Geometry: final body of the model. Coordinates: model frame, mm. Give positions to 0.01 mm unless a question says otherwise; leave off trailing zeros. Write each loop counter-clockwise with the first axis right and the second up, starting at its lowest first coordinate (ties: lowest second). Pieces come first, ordered by that corner, then holes. Notation, with made-up numbers: (48, 20) -> (98, 20) arc R24 cw to (98, 32) -> close; hole circle Ø4 at (-6.75, 88.5). An arc over 180 degrees is marked (long way). Answer as a JSON object with one key per item and string values.
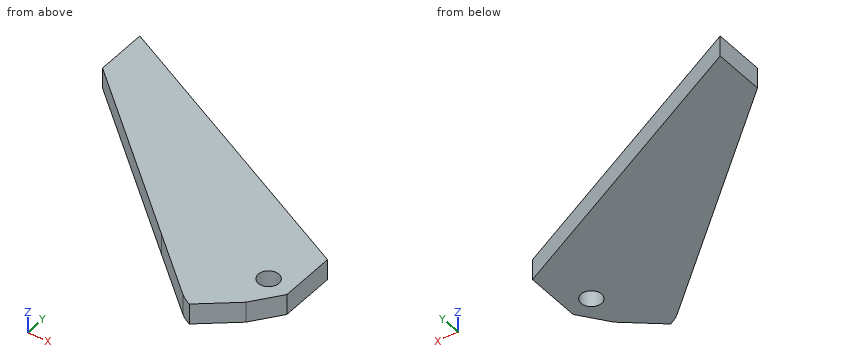
from build123d import *

# Parameters (mm, degrees)
SKETCH1_R           = 1.5
BOSS_EXTRUDE1_DEPTH = 3
CUT_EXTRUDE1_DEPTH  = 3


with BuildPart() as part:
    # Sketch1 → Boss-Extrude1 (new body)
    with BuildSketch(Plane.XY):
        with BuildLine():
            Line((2, 15), (2, 4.201633911))
            ThreePointArc((2, 4.201633911), (-1.543579693, -1.272486957), (-7.988666425, -0.280613309))
            Line((-7.988666425, -0.280613309), (-16.754941475, 7.52032788))
            Line((-16.754941475, 7.52032788), (-40.754941475, 28.877470737))
            Line((-40.754941475, 28.877470737), (-40.754941475, 36.377470737))
            Line((-40.754941475, 36.377470737), (2, 15))
        make_face()
        with Locations((-1.5, 8)):
            Circle(SKETCH1_R, mode=Mode.SUBTRACT)
    extrude(amount=BOSS_EXTRUDE1_DEPTH)

    # Sketch2 → Cut-Extrude1 (cut)
    with BuildSketch(Plane.XY.offset(3)):
        Polygon((-1.061667456, 2.832415464), (-6.529971665, -1.578677992), (-7.079129118, -3.627506614), (6.602158547, -3.973243126), (4.478348548, 4.339015555), (2, 6.845428543), align=None)
    extrude(amount=-CUT_EXTRUDE1_DEPTH, mode=Mode.SUBTRACT)


solid = part.part
Q1. Cut plane B-B (y = 8). Return the cut outline in (x, z), and give its area (3 significant figures).
Values:
{"outline": "(-17.29, 0) -> (-3, 0) -> (-3, 3) -> (-17.29, 3) -> close; (0, 0) -> (2, 0) -> (2, 3) -> (0, 3) -> close", "area": "48.9 mm²"}
Q2. Cut plane A-A (z = 2.5). Return the cut outline in (x, y).
Values:
{"outline": "(-40.75, 28.88) -> (-7.99, -0.28) arc R6 ccw to (-6.26, -1.36) -> (-1.06, 2.83) -> (2, 6.85) -> (2, 15) -> (-40.75, 36.38) -> close; hole circle Ø3 at (-1.5, 8)"}
Q3. Cut plane D-D (x = -21.5). Return the cut outline in (y, z).
Values:
{"outline": "(11.74, 0) -> (26.75, 0) -> (26.75, 3) -> (11.74, 3) -> close"}
Q4. First-contact query: P1, Ø6, axis at x = -10.5, y = 25, coming from the +Z side; P2, Ø1.5, axis at y = 5, z = 1.5, coming from the +X side. Flat tips, straight axial feed; report the tip coordinate or a pass-through.
Values:
{"P1": "through", "P2": "x = 1.16"}
Q5. Material intervals for L1, parallel to Y at x = -1.5, z = 1.4; L2, parallel to Y at x = -2.5, z = 2.3; L3, parallel to X at y = 26.5, z = 1.55, sorted ascending. Write a range as from..to.
Values:
{"L1": "2.48..6.5, 9.5..16.75", "L2": "1.67..6.88, 9.12..17.25", "L3": "-38.08..-21"}
Q6. Cut plane C-C (y = 26). Return the cut outline in (x, z).
Values:
{"outline": "(-37.52, 0) -> (-20, 0) -> (-20, 3) -> (-37.52, 3) -> close"}
